Autodesk Inventor part; units mm, degrees
ref_plane "PLATTE_XY" through (0, 0, 0) normal (0, 1, 0) x (1, 0, 0)
ref_plane "PLATTE_YZ" through (0, 0, 0) normal (1, 0, 0) x (0, 0, -1)
ref_plane "PLATTE_ZX" through (0, 0, 0) normal (0, 0, -1) x (0, 1, 0)
sketch "Sketch_1" plane through (0, 0, 0) normal (0, 1, 0) x (-1, 0, 0)
  arc A0 (125, 62.5) -> (115, 72.5) centre (115, 62.5) ccw
  line L0 (115, 72.5) -> (-115, 72.5)
  arc A1 (-115, 72.5) -> (-125, 62.5) centre (-115, 62.5) ccw
  line L1 (-125, 62.5) -> (-125, -62.5)
  arc A2 (-125, -62.5) -> (-115, -72.5) centre (-115, -62.5) ccw
  line L2 (-115, -72.5) -> (115, -72.5)
  arc A3 (115, -72.5) -> (125, -62.5) centre (115, -62.5) ccw
  line L3 (125, -62.5) -> (125, 62.5)
  circle A4 centre (-100, -47.5) radius 3.5
  circle A5 centre (-100, 47.5) radius 3.5
  circle A6 centre (-65, 0) radius 4.5
  circle A7 centre (65, 0) radius 4.5
  circle A8 centre (100, -47.5) radius 3.5
  circle A9 centre (100, 47.5) radius 3.5
extrude "Extrusion1" add sketch "Sketch_1" along normal blind 10
sketch "Sketch_9" plane through (0, 0, -32) normal (0, 0, 1) x (1, 0, 0)
  line L0 (-32, 0) -> (-32, 10)
  line L1 (-32, 10) -> (-28, 10)
  line L2 (-28, 10) -> (-28.6765, 9.3235)
  line L3 (-28.6765, 9.3235) -> (-28.6765, 0.6765)
  line L4 (-28.6765, 0.6765) -> (-28, 0)
  line L5 (-28, 0) -> (-32, 0)
  line L6 (-32, 0) -> (-32, 10)
revolve "Revolution1" cut sketch "Sketch_9" angle 360 about axis through (-32, 0, -32) along (0, -1, 0)
thread "Thread1"
sketch "Sketch_10" plane through (0, 0, -32) normal (0, 0, 1) x (1, 0, 0)
  line L0 (32, 0) -> (32, 10)
  line L1 (32, 10) -> (36, 10)
  line L2 (36, 10) -> (35.3235, 9.3235)
  line L3 (35.3235, 9.3235) -> (35.3235, 0.6765)
  line L4 (35.3235, 0.6765) -> (36, 0)
  line L5 (36, 0) -> (32, 0)
  line L6 (32, 0) -> (32, 10)
revolve "Revolution2" cut sketch "Sketch_10" angle 360 about axis through (32, 0, -32) along (0, -1, 0)
thread "Thread2"
sketch "Sketch_11" plane through (0, 0, 32) normal (0, 0, 1) x (1, 0, 0)
  line L0 (-32, 0) -> (-32, 10)
  line L1 (-32, 10) -> (-28, 10)
  line L2 (-28, 10) -> (-28.6765, 9.3235)
  line L3 (-28.6765, 9.3235) -> (-28.6765, 0.6765)
  line L4 (-28.6765, 0.6765) -> (-28, 0)
  line L5 (-28, 0) -> (-32, 0)
  line L6 (-32, 0) -> (-32, 10)
revolve "Revolution3" cut sketch "Sketch_11" angle 360 about axis through (-32, 0, 32) along (0, -1, 0)
thread "Thread3"
sketch "Sketch_12" plane through (0, 0, 32) normal (0, 0, 1) x (1, 0, 0)
  line L0 (32, 0) -> (32, 10)
  line L1 (32, 10) -> (36, 10)
  line L2 (36, 10) -> (35.3235, 9.3235)
  line L3 (35.3235, 9.3235) -> (35.3235, 0.6765)
  line L4 (35.3235, 0.6765) -> (36, 0)
  line L5 (36, 0) -> (32, 0)
  line L6 (32, 0) -> (32, 10)
revolve "Revolution4" cut sketch "Sketch_12" angle 360 about axis through (32, 0, 32) along (0, -1, 0)
thread "Thread4"
ref_plane "PLATTE_XY" through (0, 0, 0) normal (0, 1, 0) x (1, 0, 0)
ref_plane "PLATTE_YZ" through (0, 0, 0) normal (1, 0, 0) x (0, 0, -1)
ref_plane "PLATTE_ZX" through (0, 0, 0) normal (0, 0, -1) x (0, 1, 0)
properties part number "31000133platte"
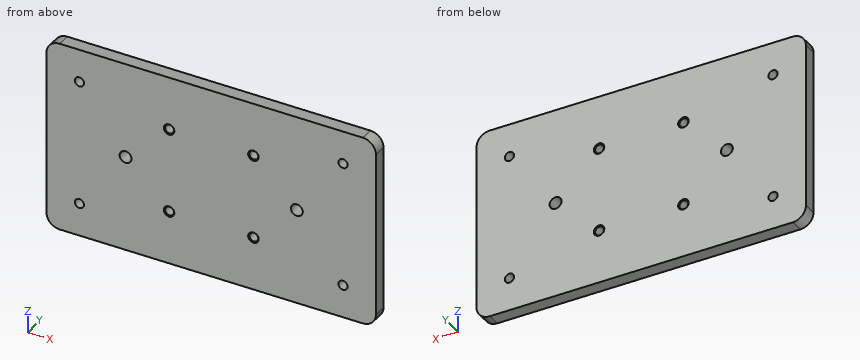
The model under review builds one solid part; all positions refer to its coordinate system, in mm. Give positions to 0.01 mm unless a question says otherwise; leave off trailing zeros. Loops run counter-clockwise (first coordinate to the right, second up) from the corner with the lowest first, then second, coordinate; pieces in that order, holes last. Notation, with made-up numbers: (-15.75, -2.75) -> (-2.75, -2.75) arc R22 ccw to (-2.75, 6.25) -> close; hole circle Ø8 at (78.25, 86). An arc over 180 degrees is marked (long way). Answer as a JSON object with one key per item and string values. Group by question number.
Q1. Insertion check: pin 1 (4 mm diameter, centred on x = -100, z = 47.5, fed in from -Y). The pin has a flat end and moves straight along its axis. Give the tip position at first contact, or say it passes through.
Q2. Take a section at B-B (z = -32). Write out the cut boundary in (x, y), plus the area to 3 significant figures.
Q3. Take a section at C-C (x = -65). Write out the cut boundary in (y, z).
Q4. Wall thickness on line 1 along Z through (x, y) = (100, 3.25); line 2 along Z through (x, y) = (-32, 5.25); line 3 along Z through (x, y) = (-65, 4): over which ranges is each line inside the solid? List them lowest first.
Q5. Take a section at D-D (x = -100). Write out the cut boundary in (y, z).
Q6. Take a section at A-A (x = -32). Write out the cut boundary in (y, z).
Answer below:
{
 "1": {"pin 1": "passes through"},
 "2": {"outline": "(-125, 0) -> (-36, 0) -> (-35.32, 0.68) -> (-35.32, 9.32) -> (-36, 10) -> (-125, 10) -> close; (-28.68, 0.68) -> (-28, 0) -> (28, 0) -> (28.68, 0.68) -> (28.68, 9.32) -> (28, 10) -> (-28, 10) -> (-28.68, 9.32) -> close; (35.32, 0.68) -> (36, 0) -> (125, 0) -> (125, 10) -> (36, 10) -> (35.32, 9.32) -> close", "area": "2,370 mm2"},
 "3": {"outline": "(0, -72.5) -> (10, -72.5) -> (10, -4.5) -> (0, -4.5) -> close; (0, 4.5) -> (10, 4.5) -> (10, 72.5) -> (0, 72.5) -> close"},
 "4": {"line 1": "z = -72.5 to -51, -44 to 44, 51 to 72.5", "line 2": "z = -72.5 to -35.32, -28.68 to 28.68, 35.32 to 72.5", "line 3": "z = -72.5 to -4.5, 4.5 to 72.5"},
 "5": {"outline": "(0, -72.5) -> (10, -72.5) -> (10, -51) -> (0, -51) -> close; (0, -44) -> (10, -44) -> (10, 44) -> (0, 44) -> close; (0, 51) -> (10, 51) -> (10, 72.5) -> (0, 72.5) -> close"},
 "6": {"outline": "(0, -72.5) -> (10, -72.5) -> (10, -36) -> (9.32, -35.32) -> (0.68, -35.32) -> (0, -36) -> close; (0, -28) -> (0.68, -28.68) -> (9.32, -28.68) -> (10, -28) -> (10, 28) -> (9.32, 28.68) -> (0.68, 28.68) -> (0, 28) -> close; (0, 36) -> (0.68, 35.32) -> (9.32, 35.32) -> (10, 36) -> (10, 72.5) -> (0, 72.5) -> close"}
}
